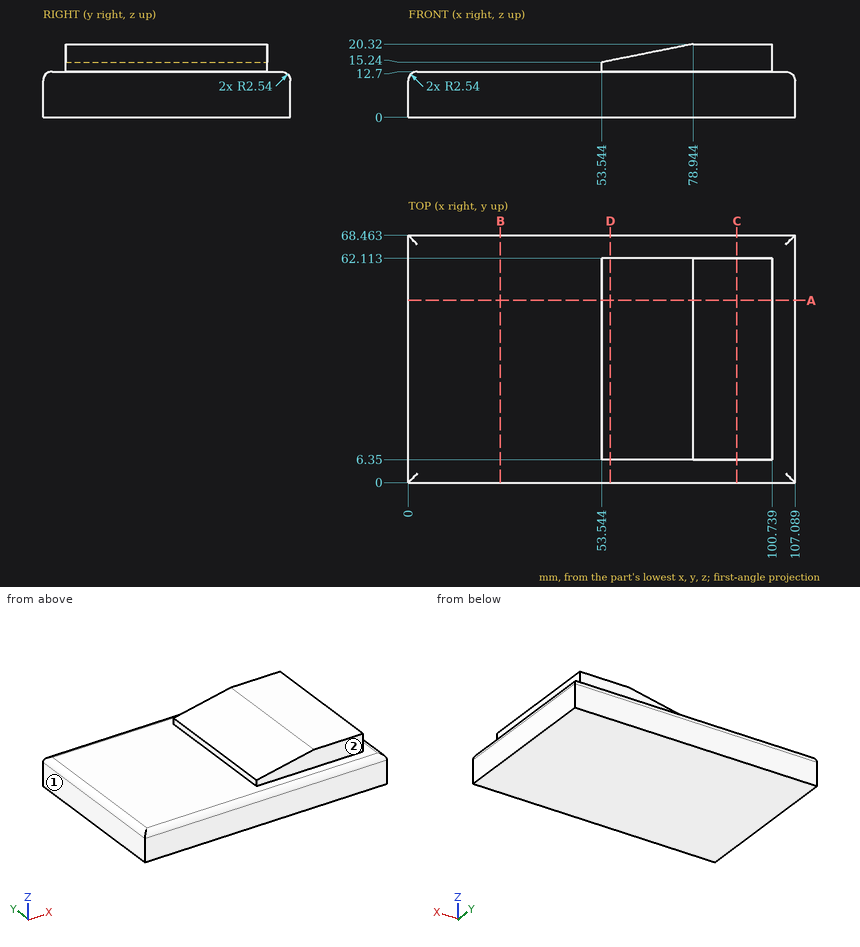
Could you check a few things on this drawing? It's one solid part, dimensions in mm from its lowest x, y, z. A direction names the side the tool comes from. Give positions to 0.01 mm unless a question says otherwise; leave off trailing zeros. Loops run counter-clockwise (first coordinate to the right, second up) from the corner with the lowest first, then second, coordinate; pieces in that order, holes last. Notation, with made-up numbers: (57.25, 76.5) -> (77.25, 76.5) arc R7 cw to (77.25, 87.5) -> close; hole circle Ø5 at (27, -33). An arc over 180 degrees is marked (long way). Use one line per item in the form item = value. Start each with the question number.
1) Imagine slicing it at C-C (x = 91). Please give me the cut outline in (y, z).
2) Imagine slicing it at A-A (y = 50.5). Please give me the cut outline in (x, z) (1 decimal).
3) Imagine slicing it at B-B (x = 25.5). Please give me the cut outline in (y, z).
4) For P1, Ø4, axis at x = 84.5, z = 16, coming from the +Y side; P2, Ø2.5, axis at x = 87.5, z = 15.5, coming from the -Y side; P3, Ø8.5, axis at y = 29.5, z = 15.5, coming from the +X side, each with a flat end and sliding along its axis, tell me the tip position at first contact or that it passes through.
5) Imagine slicing it at D-D (x = 56). Please give me the cut outline in (y, z), then the cut area to 3 significant figures.
6) Please list where these lines run through material, in increasing order: line 1 along Z through (x, y) = (11.5, 23.5); line 2 along X through (y, z) = (25, 15) (1 decimal); line 3 along Y through (x, z) = (81, 15.75).
7) Which directions (+Z, -Z, +X, -X, +Y, -Y) give clear straight access to the entire face, cutting with the end or side of a thin tool? Please do the marked faces 1 and 2.
Check values:
q1.outline = (0, 0) -> (68.46, 0) -> (68.46, 10.16) arc R2.54 ccw to (65.92, 12.7) -> (62.11, 12.7) -> (62.11, 20.32) -> (6.35, 20.32) -> (6.35, 12.7) -> (2.54, 12.7) arc R2.54 ccw to (0, 10.16) -> close
q2.outline = (0, 0) -> (107.1, 0) -> (107.1, 10.2) arc R2.5 ccw to (104.5, 12.7) -> (100.7, 12.7) -> (100.7, 20.3) -> (78.9, 20.3) -> (53.5, 15.2) -> (53.5, 12.7) -> (2.5, 12.7) arc R2.5 ccw to (0, 10.2) -> close
q3.outline = (0, 0) -> (68.46, 0) -> (68.46, 10.16) arc R2.54 ccw to (65.92, 12.7) -> (2.54, 12.7) arc R2.54 ccw to (0, 10.16) -> close
q4.P1 = 62.11
q4.P2 = 6.35
q4.P3 = 106.84
q5.outline = (0, 0) -> (68.46, 0) -> (68.46, 10.16) arc R2.54 ccw to (65.92, 12.7) -> (62.11, 12.7) -> (62.11, 15.73) -> (6.35, 15.73) -> (6.35, 12.7) -> (2.54, 12.7) arc R2.54 ccw to (0, 10.16) -> close
q5.area = 1,040 mm^2
q6.line_1 = 0 to 12.7
q6.line_2 = 53.5 to 100.7
q6.line_3 = 6.35 to 62.11
q7.face_1 = +Z, -Z, -X, +Y, -Y
q7.face_2 = +Z, +X, -X, -Y
